```python
from build123d import *

# Parameters (mm, degrees)
CIRPATTERN1_COUNT = 12


with BuildPart() as part:
    # Sketch1 → Revolve1 (revolve)
    with BuildSketch(Plane.XY, mode=Mode.PRIVATE) as revolve1_sk:
        Polygon((13.208, 43.942), (22.098, 43.942), (22.098, 41.656), (26.416, 41.656), (26.416, 43.942), (57.15, 43.942), (57.15, 38.1), (19.05, 38.1), (19.05, 0), (0, 0), (0, 43.942), (8.89, 43.942), (8.89, 41.656), (13.208, 41.656), align=None)
    revolve(revolve1_sk.sketch.rotate(Axis((0, 0, 0), (1, 0, 0)), 180), axis=Axis((0, 0, 0), (1, 0, 0)))

    # Sketch2 → 1/4-20 Tapped Hole1 (revolve, cut)
    with BuildSketch(Plane(origin=(43.18, 41.943899234, 13.099949659), x_dir=(0, -0.29811910378753365, 0.9545286794837113), z_dir=(1, 0, 0))):
        Polygon((0, 0), (0, 45.474816902), (2.5527, 43.941), (2.5527, 0), align=None)
    f_1_4_20_tapped_hole1 = revolve(axis=Axis((43.18, 48.005156349, 14.993005968), (0, -0.9545286794837113, -0.29811910378753365)), mode=Mode.SUBTRACT)

    # CirPattern1: 1/4-20 Tapped Hole1 ×12 about axis
    cirpattern1_axis = Axis((57.15, 0, 0), (-1, 0, 0))
    for i in range(1, CIRPATTERN1_COUNT):
        add(f_1_4_20_tapped_hole1.rotate(cirpattern1_axis, i * 360 / CIRPATTERN1_COUNT), mode=Mode.SUBTRACT)


solid = part.part
```
Source: CAD feature listing. Evaluate the final solid. Frame: model axes, mm. A direction names the side the tool comes from. Coordinates: 2 decimals unless noted, no trailing zeros. Loops run counter-clockwise (first coordinate to the right, second up) from the corner with the lowest first, then second, coordinate; pieces in that order, holes last. Notation, with made-up numbers: M 74.5,-38 L 93.5,-38 A33 cw 93.5,-6 Z; hole C 23.25,83.25 d9. An arc over 180 degrees is marked long. Put each result on its own line as item: value. Start each with the question number.
1) Reachability of faces 1 (the face through (24.287, -39.732, -12.512)), 2 (the face through (4.507, -41.913, -13.199)), 3 (the face through (37.83, -36.34, -11.44)) from +Z, -Z, +X, -X, +Y, -Y: full face, straight path, thin tool, end or side. Return the list, or none.
2) Ray query, L1, parallel to Z at x = 38, y = 0; L2, parallel to X at y = 23, z = 21.5; L3, parallel to Z at x = 19.5, y = -28.5. Return the intervals inside material, ascending. Write a range as from..to.
3) Contact query for flat-ended pins moving along their axis: pin 1 Ø3 at (x, z) = (40.5, -27) entering from -Y; pin 2 Ø1.5 at (y, z) = (11, 16.5) entering from +X; pin 3 Ø5 at (x, z) = (47.5, 24) entering from +Y. Output: stop coordinate, or through.
4) Cut plane A-A on y = 0. Return the cut outline in (x, z), then the cut area to 3 significant figures.
5) Pull-direction query (X, two-part tool) for faces 4 (the face through (57.15, 13, -36)), 5 (the face through (8.89, -26, -33)), 6 (the face through (45.67, 9.53, 39.9)), 7 (the face through (17.715, -41.913, -13.199)); classes: pulls with the +X half, pulls with the -X half, needs draft (parallel to the pull), parting line crosses it, or undercut.
6) Cut plane B-B on x = 39.5. Return the cut outline in (y, z).
The answers:
1. face 1: none
1. face 2: +X, -X
1. face 3: +X
2. L1: z = -43.94..-38.1, 38.1..43.94
2. L2: x = 0..19.05
2. L3: z = -33.45..-25.29, 25.29..33.45
3. pin 1: stops at y = -35.79
3. pin 2: stops at x = 19.05
3. pin 3: stops at y = 38.32
4. outline: M 0,-43.94 L 8.89,-43.94 L 8.89,-41.66 L 13.21,-41.66 L 13.21,-43.94 L 22.1,-43.94 L 22.1,-41.66 L 26.42,-41.66 L 26.42,-43.94 L 57.15,-43.94 L 57.15,-38.1 L 19.05,-38.1 L 19.05,38.1 L 57.15,38.1 L 57.15,43.94 L 26.42,43.94 L 26.42,41.66 L 22.1,41.66 L 22.1,43.94 L 13.21,43.94 L 13.21,41.66 L 8.89,41.66 L 8.89,43.94 L 0,43.94 Z
4. area: 2,080 mm²
5. face 4: pulls with the +X half
5. face 5: undercut
5. face 6: undercut
5. face 7: needs draft
6. outline: C 0,0 d87.88; hole C 0,0 d76.2
